Autodesk Fusion 360 part; units mm, degrees
sketch "Sketch1" plane through (0, 0, 0) normal (0, 0, 1) x (1, 0, 0)
  line L0 (151.5544, -62.5) -> (128.1089, -21.8911)
  line L1 (128.1089, -21.8911) -> (46.8911, 25)
  line L2 (46.8911, 25) -> (0, 25)
  line L3 (0, 0) -> (0, 25)
  arc A0 (129.9038, -75) -> (0, 0) centre (0, -150) ccw
  line L4 (151.5544, -62.5) -> (129.9038, -75)
  line L5 (113.4679, -36.5321) -> (41.5321, 5)
  line L6 (41.5321, 5) -> (0, 5)
  line L7 (134.2339, -72.5) -> (113.4679, -36.5321)
  line L8 (77.5, -15.7661) -> (87.5, 1.5544)
  point P0 (0, -150)
  point P1 (0, -150)
  dimension "d1" = 300
  dimension "d4" = 150
  dimension "d5" = 150
  dimension "d14" = 25
  dimension "d15" = 25
  dimension "d16" = 60
  dimension "d17" = 175
  dimension "d30" = 20
  dimension "d31" = 20
  dimension "d32" = 20
extrude "Extrude1" add sketch "Sketch1" along normal blind 20 contours L1 L2 L3 L5 L6 L8
mirror "Mirror2" about plane through (77.5, -15.7661, 0) normal (-0.866, 0.5, 0) of bodies 1 merged
sketch "Sketch4" plane through (0, 0, 20) normal (0, 0, 1) x (-1, 0, 0)
  line L0 (-128.1089, 21.8911) -> (-46.8911, -25)
  line L1 (-46.8911, -25) -> (0, -25)
  line L2 (-41.5321, -5) -> (-41.5321, -25) construction
  line L3 (-41.5321, -15) -> (0, -15) construction
  circle A0 centre (-7.5, -15) radius 2
  circle A1 centre (-22.5, -15) radius 2
  line L4 (-3.8, -17.1362) -> (-3.8, -12.8638)
  line L5 (-3.8, -12.8638) -> (-7.5, -10.7276)
  line L6 (-7.5, -10.7276) -> (-11.2, -12.8638)
  line L7 (-11.2, -12.8638) -> (-11.2, -17.1362)
  line L8 (-11.2, -17.1362) -> (-7.5, -19.2724)
  line L9 (-7.5, -19.2724) -> (-3.8, -17.1362)
  line L10 (-18.8, -17.1362) -> (-18.8, -12.8638)
  line L11 (-18.8, -12.8638) -> (-22.5, -10.7276)
  line L12 (-22.5, -10.7276) -> (-26.2, -12.8638)
  line L13 (-26.2, -12.8638) -> (-26.2, -17.1362)
  line L14 (-26.2, -17.1362) -> (-22.5, -19.2724)
  line L15 (-22.5, -19.2724) -> (-18.8, -17.1362)
  line L16 (0, -5) -> (-41.5321, -5)
  line L17 (-41.5321, -5) -> (-113.4679, 36.5321)
  line L18 (0, -25) -> (0, -5)
  line L19 (-113.4679, 36.5321) -> (-134.2339, 72.5)
  line L20 (-134.2339, 72.5) -> (-151.5544, 62.5)
  line L21 (-151.5544, 62.5) -> (-128.1089, 21.8911)
  line L22 (-77.5, 15.7661) -> (-87.5, -1.5544) construction
  line L23 (-142.8442, 58.8686) -> (-142.8442, 63.141)
  line L24 (-139.1442, 56.7324) -> (-142.8442, 58.8686)
  line L25 (-135.4442, 58.8686) -> (-139.1442, 56.7324)
  line L26 (-135.4442, 63.141) -> (-135.4442, 58.8686)
  line L27 (-139.1442, 65.2772) -> (-135.4442, 63.141)
  line L28 (-142.8442, 63.141) -> (-139.1442, 65.2772)
  line L29 (-131.6442, 52.2868) -> (-127.9442, 50.1506)
  line L30 (-135.3442, 50.1506) -> (-131.6442, 52.2868)
  line L31 (-135.3442, 45.8782) -> (-135.3442, 50.1506)
  line L32 (-131.6442, 43.742) -> (-135.3442, 45.8782)
  line L33 (-127.9442, 45.8782) -> (-131.6442, 43.742)
  line L34 (-127.9442, 50.1506) -> (-127.9442, 45.8782)
  circle A2 centre (-139.1442, 61.0048) radius 2
  circle A3 centre (-131.6442, 48.0144) radius 2
  point P0 (-7.5, -15)
  point P1 (-22.5, -15)
  dimension "d18" = 4
  dimension "d19" = 7.5
  dimension "d20" = 15
  dimension "d21" = 7.4
extrude "Extrude4" cut sketch "Sketch4" against normal through all contours A0 | A1 | A2 | A3
extrude "Extrude5" cut sketch "Sketch4" along normal blind 5 from surface at -20 contours L4 L5 L6 L7 L8 L9 | L10 L11 L12 L13 L14 L15
extrude "Extrude6" cut sketch "Sketch4" against normal blind 5 contours L23 L24 L25 L26 L27 L28 | L29 L30 L31 L32 L33 L34
equation "d21 = 7 mm + 2 * gap"
equation "gap = 0.2 mm"
The model under review builds one solid part; all positions refer to its coordinate system, in mm. A direction names the side the tool comes from. Round coordinates to 2 decimals unless told otherwise and drop trailing zeros. Write each loop counter-clockwise with the first axis right and the second up, starting at its lowest first coordinate (ties: lowest second). Pieces come first, ordered by that corner, then holes. Notation, with made-up numbers: M 67,-3 L 120,-3 A17 ccw 120,5 Z; hole C 78,-37.5 d5. An arc over 180 degrees is marked long. Answer as CSV lines item,"result". Start each with the question number.
Q1. Wall thickness on line 1 along Y through (x, z) = (22.5, 14); line 2 along X through (y, z) = (15, 17.25); line 3 along Y through (x, z) = (17, 17): over which ranges is each line inside the solid? List them lowest first.
Q2. Clearance check with flat-ended pins moving along their axes: P1, Ø2, axis at x = 132, y = -46.5, coming from the +Z side; P2, Ø1, axis at y = -54, z = 3, coming from the -X side; P3, Ø6.5, axis at x = 7.5, y = 15, coming from the -Z side; P4, Ø2, axis at x = 23, y = 15.5, coming from the -Z side. State where each tip first meets the part, or that it passes through.
Q3. Consider section D-D, the plane y = -0.5. Give the boundary of the cut face in (x, z).
Q4. Consider section B-B, the plane y = 15. Give the boundary of the cut face in (x, z).
Q5. Tool access review of faces 1 (the face through (129.82, -51.234, 17.535)), 2 (the face through (123.996, -54.768, 9.86)), 3 (the face through (24.376, 18.189, 2.465)): name each direction out of +Z, -Z, +X, -X, +Y, -Y from which nothing blocks a thin tool from reaching the whole face with its end or side.
Q6. The part is to be moulded in two halves that separate along Y. For faces 4 (the face through (143.015, -67.43, 9.86)), 5 (the face through (135.344, -48, 18)), 6 (the face through (22.76, 13.017, 12.605)), 7 (the face through (0, 15, 10)), say which applies: +Y half, -Y half, draft (parallel to the pull), parting line (faces both ways), or undercut.
Q7. Consider section C-C, the plane x = 102. Give the boundary of the cut face in (y, z).
Q8. Consider section A-A, the plane z = 18. Give the boundary of the cut face in (x, y).
Result set:
1,line 1,"y = 5 to 13, 17 to 25"
1,line 2,"x = 0 to 5.5, 9.5 to 20.5, 24.5 to 64.21"
1,line 3,"y = 5 to 25"
2,P1,"stops at z = 15"
2,P2,"stops at x = 123.26"
2,P3,"stops at z = 5"
2,P4,"passes through"
3,outline,"M 51.06,0 L 91.06,0 L 91.06,20 L 51.06,20 Z"
4,outline,"M 0,0 L 3.8,0 L 3.8,5 L 5.5,5 L 5.5,20 L 0,20 Z; M 9.5,5 L 11.2,5 L 11.2,0 L 18.8,0 L 18.8,5 L 20.5,5 L 20.5,20 L 9.5,20 Z; M 24.5,5 L 26.2,5 L 26.2,0 L 64.21,0 L 64.21,20 L 24.5,20 Z"
5,face 1,"+Z"
5,face 2,"+Z, -Z, -X, -Y"
5,face 3,"-Z"
6,face 4,"-Y half"
6,face 5,"undercut"
6,face 6,"undercut"
6,face 7,"draft"
7,outline,"M -29.91,0 L -6.82,0 L -6.82,20 L -29.91,20 Z"
8,outline,"M 0,5 L 41.53,5 L 77.5,-15.77 L 113.47,-36.53 L 134.23,-72.5 L 151.55,-62.5 L 128.11,-21.89 L 87.5,1.55 L 46.89,25 L 0,25 Z; hole C 7.5,15 d4; hole C 22.5,15 d4; hole M 127.94,-50.15 L 131.64,-52.29 L 135.34,-50.15 L 135.34,-45.88 L 131.64,-43.74 L 127.94,-45.88 Z; hole M 135.44,-63.14 L 139.14,-65.28 L 142.84,-63.14 L 142.84,-58.87 L 139.14,-56.73 L 135.44,-58.87 Z"
